Input: part model. Units: mm. Frame: model coordinates. Round coordinates to 2 decimals unless told otherwise and drop trailing zeros. Loops run counter-clockwise (first coordinate to the right, second up) from the corner with the lowest first, then second, coordinate; pieces in that order, holes last. Notation, with made-up numbers: M -5.5,75.5 L 49.5,75.5 A29 ccw 49.5,110.5 Z; hole C 82,-31 d5. An arc over 180 degrees is marked long. Return JSON: item names as keys, results as strings. Group by question number.
1) Section B-B (y = 2.25). Output: boundary loops of the cut face in (x, z).
2) Section D-D (z = 8.5). Output: boundary loops of the cut face in (x, y).
3) Material intervals for line 1 (X direction, y = 4.35, z = 8.5); line 2 (Z direction, x = -49.75, y = 2.5); line 3 (Z direction, x = -42.5, y = 5), sorted ascending. Write a range as from..to.
4) Section C-C (x = -49.75). Output: boundary loops of the cut face in (y, z).
5) Section A-A (z = -5.5). Output: boundary loops of the cut face in (x, y).
Autodesk Inventor part; units mm, degrees
ref_plane "YZ Plane" through (0, 0, 0) normal (1, 0, 0) x (0, 1, 0)
ref_plane "XZ Plane" through (0, 0, 0) normal (0, 1, 0) x (-1, 0, 0)
ref_plane "XY Plane" through (0, 0, 0) normal (0, 0, 1) x (1, 0, 0)
sketch "Sketch1" plane through (0, 0, 0) normal (0, 1, 0) x (-1, 0, 0)
  line L0 (0, 0) -> (-16.25, 0)
  line L1 (0, 0) -> (46.75, 0)
  line L2 (300, 0) -> (330, 0) construction
  line L3 (330, 30) -> (-30, 30) construction
  line L4 (-16.25, 15.5) -> (46.75, 15.5)
  line L5 (46.75, 15.5) -> (46.75, 0)
  line L6 (46.75, -15.5) -> (-16.25, -15.5)
  line L7 (-16.25, -15.5) -> (-16.25, 0)
  line L8 (-16.25, 15.5) -> (46.75, -15.5) construction
  line L9 (46.75, 15.5) -> (-16.25, -15.5) construction
  line L10 (-19.25, 8.5) -> (49.75, 8.5) construction
  line L11 (49.75, 8.5) -> (49.75, -8.5) construction
  line L12 (49.75, -8.5) -> (-19.25, -8.5) construction
  line L13 (-19.25, -8.5) -> (-19.25, 8.5) construction
  line L14 (-19.25, 8.5) -> (49.75, -8.5) construction
  line L15 (49.75, 8.5) -> (-19.25, -8.5) construction
  line L16 (-30, 0) -> (-30, 30)
  line L17 (330, 0) -> (330, 30) construction
  line L18 (46.75, 0) -> (300, 0) construction
  line L19 (46.75, 0) -> (46.75, -15.5)
  line L20 (-16.25, 0) -> (-30, 0)
  line L21 (-16.25, 0) -> (-16.25, 15.5)
  line L22 (300, 0) -> (300, 18.5) construction
  line L23 (0, 0) -> (-30, 0) construction
  line L24 (46.75, 0) -> (61.75, 0)
  line L25 (61.75, 0) -> (61.75, 30)
  line L26 (-30, 30) -> (61.75, 30)
  point P0 (15.25, 0)
  point P1 (15.25, 0)
  point P2 (285, 0)
  dimension "d0" = 300
  dimension "d5" = 63
  dimension "d6" = 31
  dimension "d7" = 69
  dimension "d8" = 17
  dimension "d9" = 16.25
  dimension "d10" = 30
  dimension "d11" = 30
  dimension "d20" = 18.5
  dimension "d21" = 15
  dimension "d29" = 15
extrude "Extrusion1" add sketch "Sketch1" along normal blind 6 contours L20 L16 L26 L25 L24 L5 L4 L21
hole "Hole1" at (19.25, 0, 8.5) at (-49.75, 0, 8.5) direction (0, 1, 0) diameter 2 end through all
fillet "Fillet1" radius 20 1 edges at (30, 3, 30)
mirror "Mirror1" about plane through (30, 0, 0) normal (0, 0, -1)
properties part number "segment1c" material "Plywood, Finish"
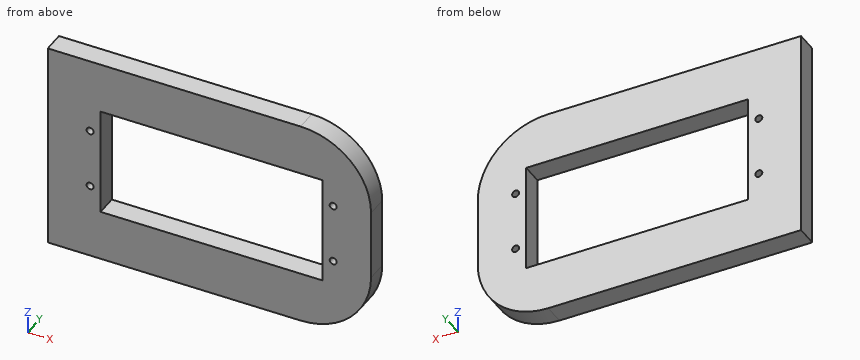
Returned:
{
 "1": {"outline": "M -61.75,-30 L 10,-30 A20 ccw 30,-10 L 30,10 A20 ccw 10,30 L -61.75,30 Z; hole C -49.75,-8.5 d2; hole C -49.75,8.5 d2; hole M -46.75,-15.5 L 16.25,-15.5 L 16.25,15.5 L -46.75,15.5 Z; hole C 19.25,-8.5 d2; hole C 19.25,8.5 d2"},
 "2": {"outline": "M -61.75,0 L -50.75,0 L -50.75,6 L -61.75,6 Z; M -48.75,0 L -46.75,0 L -46.75,6 L -48.75,6 Z; M 16.25,0 L 18.25,0 L 18.25,6 L 16.25,6 Z; M 20.25,0 L 30,0 L 30,6 L 20.25,6 Z"},
 "3": {"line 1": "x = -61.75..-50.75, -48.75..-46.75, 16.25..18.25, 20.25..30", "line 2": "z = -30..-9.5, -7.5..7.5, 9.5..30", "line 3": "z = -30..-15.5, 15.5..30"},
 "4": {"outline": "M 0,-30 L 6,-30 L 6,-9.5 L 0,-9.5 Z; M 0,-7.5 L 6,-7.5 L 6,7.5 L 0,7.5 Z; M 0,9.5 L 6,9.5 L 6,30 L 0,30 Z"},
 "5": {"outline": "M -61.75,0 L -46.75,0 L -46.75,6 L -61.75,6 Z; M 16.25,0 L 30,0 L 30,6 L 16.25,6 Z"}
}
